Can you work these out from the model? Positions are in its coordinate system, mm. A direction names the side the tool comes from. Coordinates: 2 decimals unless noted, no trailing zeros. Order: outer loops, then holes, each group sorted by start corner. A loop starts at its lowest first (then second) coordinate and runs counter-clockwise, first axis right, second up. Notation, with made-up numbers: (-11.5, 76) -> (-2.5, 76) arc R26 ccw to (-2.5, 102) -> close; hole circle Ø10 at (85.25, -32.75). An arc over 180 degrees is marked (long way). Answer as CSV lines item,"result".
from build123d import *

# Parameters (mm, degrees)
SKETCH005_R   = 2
SKETCH005_R_2 = 2.65
PAD_DEPTH     = 4
FILLET_R      = 15
FILLET001_R   = 7
FILLET002_R   = 7
FILLET003_R   = 1


with BuildPart() as part:
    # Sketch005 → Pad (new body)
    with BuildSketch(Plane.XY.offset(-3)):
        Polygon((-38, 10), (-31, 10), (-31, -10), (9, -10), (9, 10), (17, 10), (47, 0.7), (47, -9.185045), (30, -19), (-35, -19), (-50, -10.339746), (-50, 3.07), align=None)
        with Locations((-35.5, 5)):
            Circle(SKETCH005_R, mode=Mode.SUBTRACT)
        with Locations((-35.5, -5)):
            Circle(SKETCH005_R, mode=Mode.SUBTRACT)
        with Locations((13.5, 5)):
            Circle(SKETCH005_R, mode=Mode.SUBTRACT)
        with Locations((13.5, -5)):
            Circle(SKETCH005_R, mode=Mode.SUBTRACT)
        with Locations((-44.5, 0)):
            Circle(SKETCH005_R_2, mode=Mode.SUBTRACT)
        with Locations((40.5, -5)):
            Circle(SKETCH005_R_2, mode=Mode.SUBTRACT)
    extrude(amount=PAD_DEPTH)

    # Fillet
    fillet_edges = [part.edges().sort_by_distance(p)[0] for p in [
        (30, -19, -1),
        (-35, -19, -1),
    ]]
    fillet(fillet_edges, radius=FILLET_R)

    # Fillet001
    fillet001_edges = [part.edges().sort_by_distance(p)[0] for p in [
        (-50, -10.339746, -1),
        (47, -9.185045, -1),
    ]]
    fillet(fillet001_edges, radius=FILLET001_R)

    # Fillet002
    fillet002_edges = [part.edges().sort_by_distance(p)[0] for p in [
        (-50, 3.07, -1),
        (-38, 10, -1),
        (17, 10, -1),
        (47, 0.7, -1),
    ]]
    fillet(fillet002_edges, radius=FILLET002_R)

    # Fillet003
    fillet003_edges = [part.edges().sort_by_distance(p)[0] for p in [
        (-31, 10, -1),
        (9, 10, -1),
        (9, -10, -1),
        (-31, -10, -1),
    ]]
    fillet(fillet003_edges, radius=FILLET003_R)


solid = part.part
Q1. Which directions (+Z, -Z, +X, -X, +Y, -Y) give clear straight access to the entire face, cutting with the end or side of a thin tool? Please do faces 1 (the flat face through (13, 10, -1)), 2 (the flat face through (-31, 0, -1)).
Solution:
face 1,"+Z, -Z, +X, -X, +Y"
face 2,"+Z, -Z, +Y"
Q2. Imagine slicing it at A-A (x = 13.5). List the corners of the cut face in (y, z) for me.
Solution:
outline,"(-19, -3) -> (-7, -3) -> (-7, 1) -> (-19, 1) -> close; (-3, -3) -> (3, -3) -> (3, 1) -> (-3, 1) -> close; (7, -3) -> (10, -3) -> (10, 1) -> (7, 1) -> close"
Q3. For P1, Ø2.5, axis at x = 13.5, y = 5, coming from the +Z side, with a flat end and sliding along its axis, tell me the tip position at first contact or that it passes through.
Solution:
P1,"through"
Q4. Imagine slicing it at B-B (z = -2.1). Give the number of separate pieces and of enclosed holes in the cut face, and give its area (3 significant figures).
Solution:
separate pieces,"1"
enclosed holes,"6"
area,"1,570 mm2"
Q5. Imagine slicing it at C-C (y = 4). List the corners of the cut face in (x, z) for me.
Solution:
outline,"(-47.93, -3) -> (-37.23, -3) -> (-37.23, 1) -> (-47.93, 1) -> close; (-33.77, -3) -> (-31, -3) -> (-31, 1) -> (-33.77, 1) -> close; (9, -3) -> (11.77, -3) -> (11.77, 1) -> (9, 1) -> close; (15.23, -3) -> (36.35, -3) -> (36.35, 1) -> (15.23, 1) -> close"
Q6. If I drill on line 1 (Y direction, x = 13.5, z = -0.35); line 2 (X direction, y = 0.75, z = 0.25); line 3 (X direction, y = -6.5, z = -1.85), over which ranges is the centre line in solid material (lowest first)?
Solution:
line 1,"-19 to -7, -3 to 3, 7 to 10"
line 2,"-49.79 to -47.04, -41.96 to -31, 9 to 44.68"
line 3,"-50 to -36.82, -34.18 to -31, 9 to 12.18, 14.82 to 38.32, 42.68 to 46.87"
Q7. Imagine slicing it at D-D (x = -44.5). List the corners of the cut face in (y, z) for me, and give its area (3 significant figures).
Solution:
outline,"(-13.52, -3) -> (-2.65, -3) -> (-2.65, 1) -> (-13.52, 1) -> close; (2.65, -3) -> (6.25, -3) -> (6.25, 1) -> (2.65, 1) -> close"
area,"57.8 mm2"
Q8. We'd pull the mould along X, two halves only. Please class faces 3 (the flat face through (29.9, 6, -1)), 4 (the flat face through (-43.11, 7.05, -1.03)), 5 (the flat face through (-11, -10, -1)): pulls with the +X half, pulls with the -X half, needs draft (parallel to the pull), parting line crosses it, or undercut.
Solution:
face 3,"pulls with the +X half"
face 4,"pulls with the -X half"
face 5,"undercut"
